```python
from build123d import *

# Parameters (mm, degrees)
SKETCH1_R           = 55
BOSS_EXTRUDE1_DEPTH = 2
SKETCH2_R           = 2
CUT_EXTRUDE1_DEPTH  = 0.25
SKETCH3_R           = 34
CUT_EXTRUDE2_DEPTH  = 10


with BuildPart() as part:
    # Sketch1 → Boss-Extrude1 (new body)
    with BuildSketch(Plane(origin=(0, 0, 0), x_dir=(1, 0, 0), z_dir=(0, 1, 0))):
        Circle(SKETCH1_R)
    extrude(amount=BOSS_EXTRUDE1_DEPTH)

    # Sketch2 → Cut-Extrude1 (cut)
    with BuildSketch(Plane(origin=(0, 2, 0), x_dir=(1, 0, 0), z_dir=(0, 1, 0))):
        with Locations((0, 44.5)):
            Circle(SKETCH2_R)
        with Locations((44.5, 0)):
            Circle(SKETCH2_R)
        with Locations((0, -44.5)):
            Circle(SKETCH2_R)
        with Locations((-44.5, 0)):
            Circle(SKETCH2_R)
    extrude(amount=-CUT_EXTRUDE1_DEPTH, mode=Mode.SUBTRACT)

    # Sketch3 → Cut-Extrude2 (cut)
    with BuildSketch(Plane(origin=(0, 2, 0), x_dir=(1, 0, 0), z_dir=(0, 1, 0))):
        Circle(SKETCH3_R)
    extrude(amount=-CUT_EXTRUDE2_DEPTH, mode=Mode.SUBTRACT)


solid = part.part
```
Verification items for the finished model (mm, model axes). A direction names the side the tool comes from. Coordinates: 2 decimals unless noted, no trailing zeros. Order: outer loops, then holes, each group sorted by start corner. A loop starts at its lowest first (then second) coordinate and runs counter-clockwise, first axis right, second up. Notation, with made-up numbers: (35, 73.25) -> (53, 73.25) arc R23 cw to (53, 92.25) -> close; hole circle Ø10 at (-38, -10.5). An arc over 180 degrees is marked (long way). Answer as CSV lines item,"result". Start each with the question number.
1) Cross-section at D-D, the plane z = -5. Record the boundary of the cut face in (x, y).
2) Cross-section at A-A, the plane x = 0. Record the boundary of the cut face in (y, z).
3) Material ranges on L1, parallel to X at y = 1.9, z = 0; L2, parallel to Z at x = 0, y = 0.75, recorded low to high. Write a range as [from, to].
4) Gauge pin test, flat end, axial feed: pin 1 Ø2.5 at (x, z) = (0, 44.5) entering from +Y. Record the tip position at first contact, or that the pin passes through.
5) Set-up check for faces 4 (the face through (0, 1.75, 44)), 5 (the face through (-25, 0, 24)): record each of +Z, -Z, +X, -X, +Y, -Y from which the full face is reachable in a straight line by a thin tool's end or side.
6) Cross-section at C-C, the plane y = 0.5. Record the boundary of the cut face in (x, z), then the cut area to 3 significant figures.
7) Release check for a two-part mould opening along Z. For faces 1 (the face through (-11.923, 0.986, 53.692)), 2 (the face through (0, 1.75, -45)), 3 (the face through (-25, 2, 24)) record: released by +Z, released by -Z, zero draft, split by the parting line, or undercut.
8) Cross-section at B-B, the plane z = 17. Record the boundary of the cut face in (x, y), then the cut area to 3 significant figures.
Conclusion:
1,outline,"(-54.77, 0) -> (-33.63, 0) -> (-33.63, 2) -> (-54.77, 2) -> close; (33.63, 0) -> (54.77, 0) -> (54.77, 2) -> (33.63, 2) -> close"
2,outline,"(0, -55) -> (2, -55) -> (2, -46.5) -> (1.75, -46.5) -> (1.75, -42.5) -> (2, -42.5) -> (2, -34) -> (0, -34) -> close; (0, 34) -> (2, 34) -> (2, 42.5) -> (1.75, 42.5) -> (1.75, 46.5) -> (2, 46.5) -> (2, 55) -> (0, 55) -> close"
3,L1,"x = [-55, -46.5], [-42.5, -34], [34, 42.5], [46.5, 55]"
3,L2,"z = [-55, -34], [34, 55]"
4,pin 1,"stops at y = 1.75"
5,face 4,"+Y"
5,face 5,"+Z, -Z, +X, -X, -Y"
6,outline,"circle Ø110 at (0, 0); hole circle Ø68 at (0, 0)"
6,area,"5,870 mm²"
7,face 1,"split by the parting line"
7,face 2,"undercut"
7,face 3,"zero draft"
8,outline,"(-52.31, 0) -> (-29.44, 0) -> (-29.44, 2) -> (-52.31, 2) -> close; (29.44, 0) -> (52.31, 0) -> (52.31, 2) -> (29.44, 2) -> close"
8,area,"91.4 mm²"
